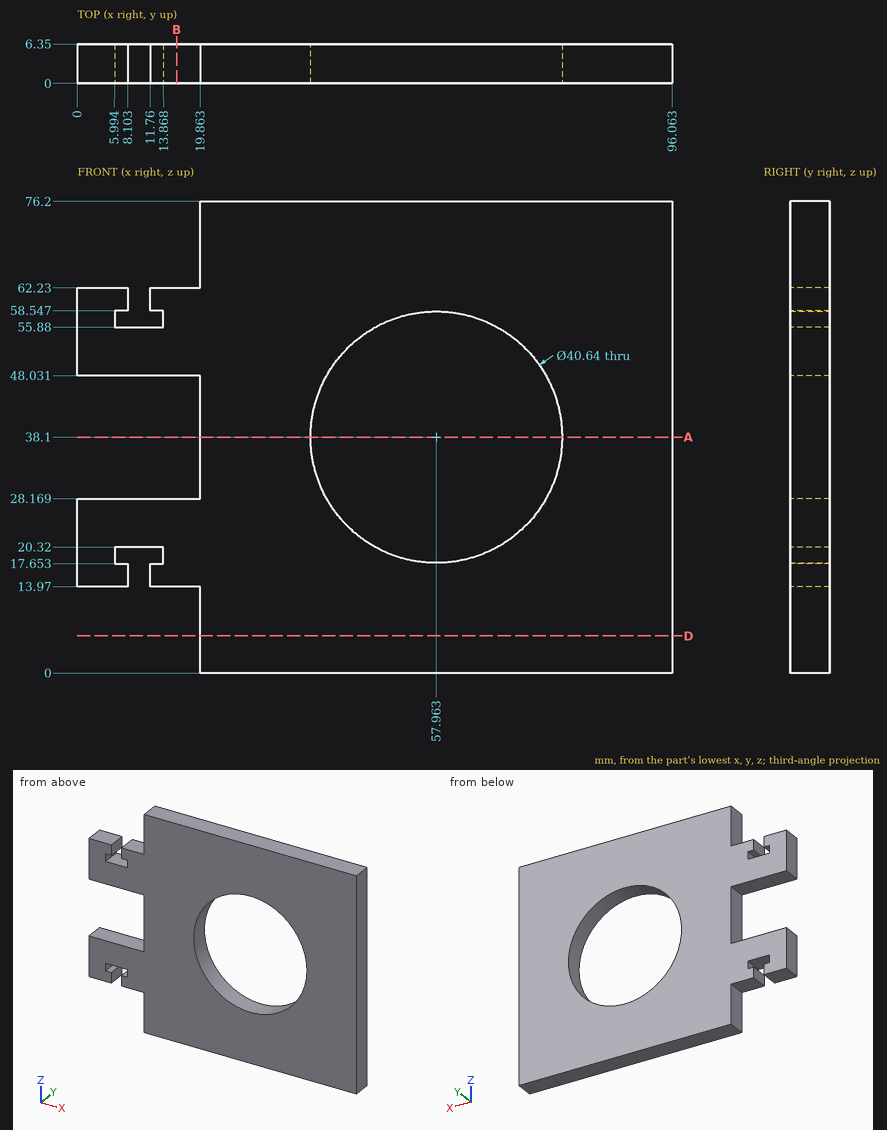
Part print with two shaded views. Sizes in mm from the minimum x, y, z corner. Round coordinates to 2 decimals unless told otherwise and drop trailing zeros. Write each loop counter-clockwise with the first axis right and the second up, starting at its lowest first coordinate (ties: lowest second). Pieces come first, ordered by that corner, then holes. Notation, with made-up numbers: (52.5, 11.5) - (57.5, 11.5) arc R27 ccw to (57.5, 44.5) - close; hole circle Ø5 at (14.25, 79.5). An arc over 180 degrees is marked (long way). Answer as CSV lines item,"result".
Q1. Cut at D-D (z = 6). Write the cut outline in (x, y).
Report:
outline,"(19.86, 0) - (96.06, 0) - (96.06, 6.35) - (19.86, 6.35) - close"
Q2. Cut at B-B (x = 16). Write the cut outline in (y, z), and give its area (3 significant figures).
Report:
outline,"(0, 13.97) - (6.35, 13.97) - (6.35, 28.17) - (0, 28.17) - close; (0, 48.03) - (6.35, 48.03) - (6.35, 62.23) - (0, 62.23) - close"
area,"180 mm^2"
Q3. Drop flat-ended pins along their axis: pin 1 (1.9 mm diameter, centred on x = 18, y = 2.5, fed in from -Z); pin 2 (1.1 mm diameter, centred on x = 7.5, y = 4.5, fed in from +Z); pin 3 (3 mm diameter, centred on y = 4, z = 10.5, fed in from -X). Give the stop position or say it passes through.
Report:
pin 1,"stops at z = 13.97"
pin 2,"stops at z = 62.23"
pin 3,"stops at x = 19.86"
Q4. Drill centre lines: probe 1 along X at (y, z) = (4.25, 38.1); probe 2 along Z at (x, y) = (19, 3.75); probe 3 along Z at (x, y) = (40.5, 1.25). Where is each one in solid material? Low to high. Write a range as [from, to].
Report:
probe 1,"x = [19.86, 37.64], [78.28, 96.06]"
probe 2,"z = [13.97, 28.17], [48.03, 62.23]"
probe 3,"z = [0, 27.71], [48.49, 76.2]"
Q5. Cut at A-A (z = 38.1). Write the cut outline in (x, y), and give its area (3 significant figures).
Report:
outline,"(19.86, 0) - (37.64, 0) - (37.64, 6.35) - (19.86, 6.35) - close; (78.28, 0) - (96.06, 0) - (96.06, 6.35) - (78.28, 6.35) - close"
area,"226 mm^2"
